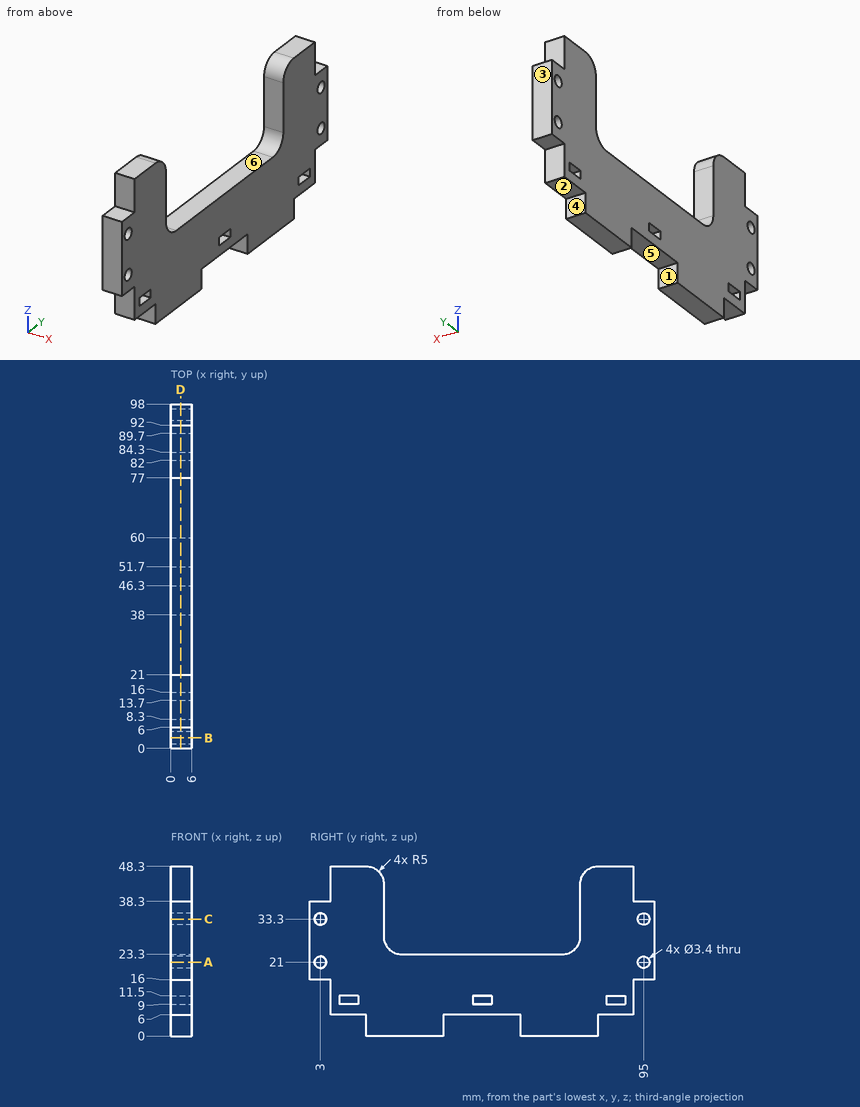
Study the drawing (mm; zero at the part's minimum x, y, z) and answer. A direction names the side the tool comes from. Give positions to 0.01 mm unless a question says otherwise; leave off trailing zeros. Loops run counter-clockwise (first coordinate to the right, second up) from the corner with the lowest first, then second, coordinate; pieces in that order, holes last. Notation, with made-up numbers: M 47.5,86 L 106.5,86 A17 cw 106.5,116 Z; hole C -21.75,61 d1. An arc over 180 degrees is marked long. Use CSV: the item, a comma, the result in double quotes.
1) Find section B-B on y = 3. Write down the section's boundary in (x, z), plus the area to 3 significant figures.
Answer:
outline,"M 0,16 L 6,16 L 6,19.3 L 0,19.3 Z; M 0,22.7 L 6,22.7 L 6,31.6 L 0,31.6 Z; M 0,35 L 6,35 L 6,38.3 L 0,38.3 Z"
area,"93.0 mm^2"
2) Find section D-D on x = 2.8. Give the number of separate pieces and of enclosed holes in the cut face, plus the area to 3 significant figures.
Answer:
separate pieces,"1"
enclosed holes,"7"
area,"2,690 mm^2"
3) Consider L1, parallel to Z at x = 3.7, y = 95; L2, parallel to Y at x = 2.6, z = 21; L3, parallel to Y at x = 3.05, z = 40. Determine where each line is inside the solid, lowest interval first.
Answer:
L1,"16 to 19.3, 22.7 to 31.6, 35 to 38.3"
L2,"0 to 1.3, 4.7 to 93.3, 96.7 to 98"
L3,"6 to 21, 77 to 92"
4) Determine the mould class of the marked faces 1, 2 and 3 for opening direction Y: released by +Y, released by -Y, zero draft, split by the parting line, or undercut.
Answer:
face 1,"undercut"
face 2,"zero draft"
face 3,"released by +Y"
5) Find section C-C on z = 33.3. Write down the section's boundary in (x, y).
Answer:
outline,"M 0,0 L 6,0 L 6,1.3 L 0,1.3 Z; M 0,4.7 L 6,4.7 L 6,21 L 0,21 Z; M 0,77 L 6,77 L 6,93.3 L 0,93.3 Z; M 0,96.7 L 6,96.7 L 6,98 L 0,98 Z"
6) Given P1, Ø2, axis at x = 4.5, z = 10, coming from the +Y side; P2, Ø2, axis at x = 3.5, y = 52, coming from the +Z side; P3, Ø2, axis at x = 4, z = 10.5, coming from the -Y side, each flat-ended and moving along its own axis, determine where each tip first touches the part or whether it passes through.
Answer:
P1,"y = 92"
P2,"z = 23.3"
P3,"y = 6"
7) Find section A-A on z = 21. Write down the section's boundary in (x, y).
Answer:
outline,"M 0,0 L 6,0 L 6,1.3 L 0,1.3 Z; M 0,4.7 L 6,4.7 L 6,93.3 L 0,93.3 Z; M 0,96.7 L 6,96.7 L 6,98 L 0,98 Z"
8) Which of the six approach directions +Z, -Z, +X, -X, +Y, -Y give full straight-line access (tool end or side, diameter ignored) to the marked faces 4, 5 and 6?
Answer:
face 4,"-Z, +X, -X, +Y"
face 5,"-Z, +X, -X"
face 6,"+Z, +X, -X"
